```python
from build123d import *

# Parameters (mm, degrees)
CROQUIS2_R                             = 5
SALIENTE_EXTRUIR1_DEPTH                = 60
CROQUIS3_R                             = 7
SALIENTE_EXTRUIR2_DEPTH                = 2
CORTAR_EXTRUIR1_REACH                  = 64.785
CORTAR_EXTRUIR1_END_RADIUS             = 5
CROQUIS4_R                             = 1
CORTAR_EXTRUIR1_DIRECTION_2_REACH      = 64.785
CORTAR_EXTRUIR1_DIRECTION_2_END_RADIUS = 5


with BuildPart() as part:
    # Croquis2 → Saliente-Extruir1 (new body)
    with BuildSketch(Plane(origin=(0, 0, 0), x_dir=(1, 0, 0), z_dir=(0, 1, 0))):
        with Locations(Location((0, 0, 0), (0, 0, 270))):
            Circle(CROQUIS2_R)
    extrude(amount=SALIENTE_EXTRUIR1_DEPTH)

    # Croquis3 → Saliente-Extruir2 (add)
    with BuildSketch(Plane(origin=(0, 60, 0), x_dir=(1, 0, 0), z_dir=(0, 1, 0))):
        with Locations(Location((0, 0, 0), (0, 0, 270))):
            Circle(CROQUIS3_R)
    extrude(amount=SALIENTE_EXTRUIR2_DEPTH)

    # Cortar-Extruir1: up to this cylinder (the profile starts inside it)
    cortar_extruir1_end = Plane(origin=(0, 2, 0), z_dir=(0, -1, 0)) * Cylinder(CORTAR_EXTRUIR1_END_RADIUS, 140.57, mode=Mode.PRIVATE)
    # Croquis4 → Cortar-Extruir1 (cut, up to the surface)
    with BuildSketch(Plane.XY, mode=Mode.PRIVATE) as cortar_extruir1_sk1:
        with Locations((0, 2)):
            Circle(CROQUIS4_R)
    cortar_extruir1_tool1 = extrude(cortar_extruir1_sk1.sketch, amount=-CORTAR_EXTRUIR1_REACH, mode=Mode.PRIVATE) & cortar_extruir1_end
    add(cortar_extruir1_tool1.solids().sort_by_distance((0, 2, 0))[0], mode=Mode.SUBTRACT)

    # Cortar-Extruir1 direction 2: up to this cylinder (the profile starts inside it)
    cortar_extruir1_direction_2_end = Plane(origin=(0, 2, 0), z_dir=(0, -1, 0)) * Cylinder(CORTAR_EXTRUIR1_DIRECTION_2_END_RADIUS, 140.57, mode=Mode.PRIVATE)
    # Croquis4 → Cortar-Extruir1 direction 2 (cut, up to the surface)
    with BuildSketch(Plane.XY, mode=Mode.PRIVATE) as cortar_extruir1_direction_2_sk1:
        with Locations((0, 2)):
            Circle(CROQUIS4_R)
    cortar_extruir1_direction_2_tool1 = extrude(cortar_extruir1_direction_2_sk1.sketch, amount=CORTAR_EXTRUIR1_DIRECTION_2_REACH, mode=Mode.PRIVATE) & cortar_extruir1_direction_2_end
    add(cortar_extruir1_direction_2_tool1.solids().sort_by_distance((0, 2, 0))[0], mode=Mode.SUBTRACT)


solid = part.part
```
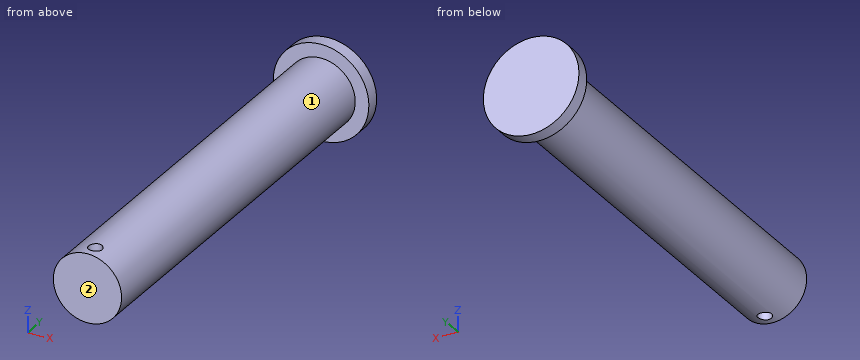
The model under review builds one solid part; all positions refer to its coordinate system, in mm. Face numbers are marked on the shaded views. A direction names the side the tool comes from. Round coordinates to 2 decimals unless told otherwise and drop trailing zeros. Loops run counter-clockwise (first coordinate to the right, second up) from the corner with the lowest first, then second, coordinate; pieces in that order, holes last. Notation, with made-up numbers: (64.5, 9.25) - (123.5, 9.25) arc R22 ccw to (123.5, 32.25) - close; hole circle Ø9 at (-20.75, 42). An arc over 180 degrees is marked (long way). Use a Markdown table: item, result. Add a question column.
Q1. Add section D-D (y = 2). State the section outline as (x, z) points, plus the area to 3 significant figures.
Q2. Add section C-C (x = 3). State the section outline as (y, z) points, plus the area to 3 significant figures.
Q3. For probe 1 along X at (y, z) = (2, 0.25); probe 2 along Y at (x, z) = (0, -1.5); probe 3 along X at (y, z) = (52.5, 0), list the stretches that pass through material, from the lowest coordinate up.
Q4. Insertion check: pin 1 Ø8 at (x, y) = (1, 39.5) entering from -Z; pin 2 Ø4 at (x, y) = (4.5, 38.5) entering from +Z; pin 3 Ø5 at (y, z) = (29, -5) entering from +X. Each pin has a flat end and moves straight along its axis. Give the tip position at first contact, or say it passes through.
Q5. Add section B-B (z = 4). State the section outline as (x, y) points.
Q6. Add section A-A (x = 0). State the section outline as (y, z) points.
Q7. Machinability: for the marked faces 1 and 2, which of the approach directions +Z, -Z, +X, -X, +Y, -Y give a long, thin tool a straight path to every point of the face, cutting with its end or side? Answer none if there is none.
Worked answers:
| question | item | result |
|---|---|---|
| 1 | outline | (-1, -4.9) - (-1, 4.9) arc R5 ccw to start; (1, -4.9) arc R5 ccw to (1, 4.9) - close |
| 1 | area | 58.7 mm² |
| 2 | outline | (0, -4) - (60, -4) - (60, -6.32) - (62, -6.32) - (62, 6.32) - (60, 6.32) - (60, 4) - (0, 4) - close |
| 2 | area | 505 mm² |
| 3 | probe 1 | -4.99 to -1, 1 to 4.99 |
| 3 | probe 2 | 0 to 1, 3 to 62 |
| 3 | probe 3 | -5 to 5 |
| 4 | pin 1 | z = -5 |
| 4 | pin 2 | z = 4.33 |
| 4 | pin 3 | x = 4.33 |
| 5 | outline | (-5.74, 60) - (-3, 60) - (-3, 0) - (3, 0) - (3, 60) - (5.74, 60) - (5.74, 62) - (-5.74, 62) - close; hole circle Ø2 at (0, 2) |
| 6 | outline | (0, -5) - (1, -5) - (1, 5) - (0, 5) - close; (3, -5) - (60, -5) - (60, -7) - (62, -7) - (62, 7) - (60, 7) - (60, 5) - (3, 5) - close |
| 7 | face 1 | -Y |
| 7 | face 2 | +Z, -Z, +X, -X, -Y |
